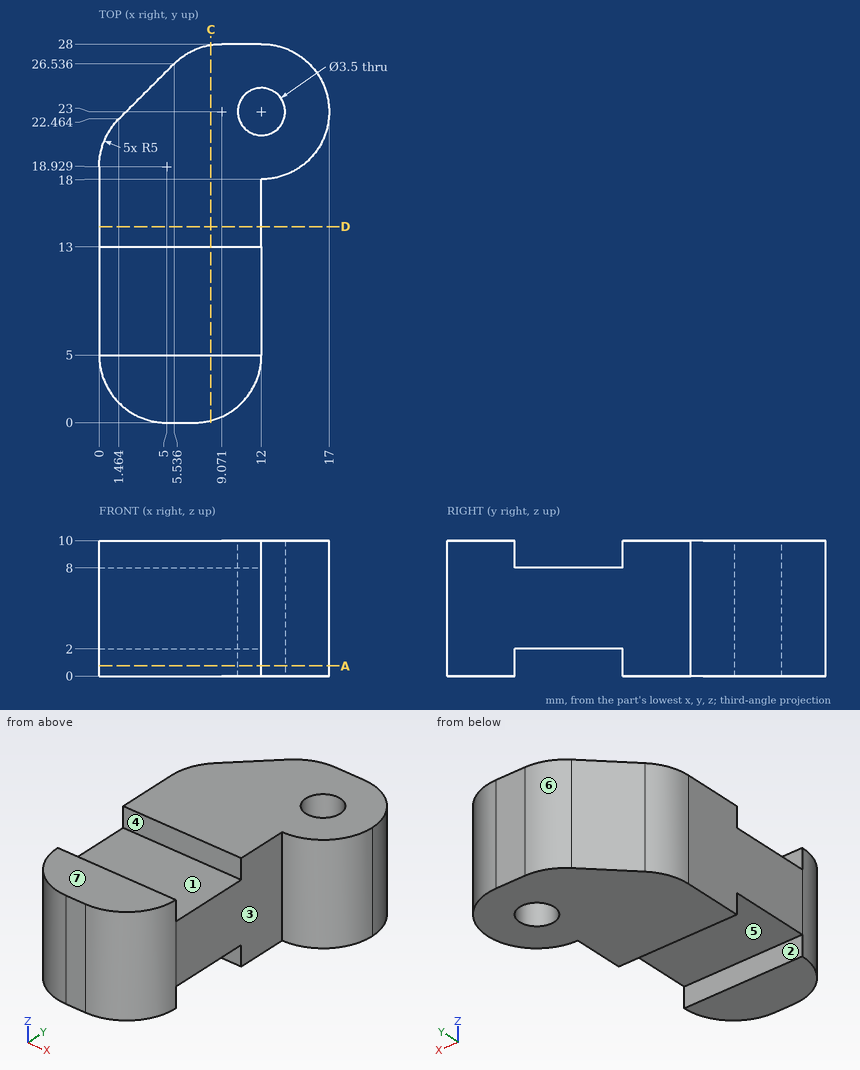
The figure shows three views and two pictorial views of one solid part (mm, origin at its lowest corner). Answer the questions. A direction names the side the tool comes from. Round coordinates to 2 decimals unless told otherwise and drop trailing zeros. Write each loop counter-clockwise with the first axis right and the second up, starting at its lowest first coordinate (ties: lowest second). Pieces come first, ordered by that corner, then holes. Notation, with made-up numbers: M 27.5,1.25 L 67.5,1.25 A35 ccw 67.5,39.25 Z; hole C -22,2.25 d4. An arc over 180 degrees is marked long. Use a Markdown table: item, result.
1) Consider line 1 (X direction, y = 10.25, z = 7.75); line 2 (Z direction, x = 6.25, y = 7.5); line 3 (X direction, y = 23.5, z = 7.25) (1 decimal). Determine where each line is inside the solid, lowest interval first. Write a range as [from, to].
Taken from the geometry:
| item | result |
|---|---|
| line 1 | x = [0, 12] |
| line 2 | z = [2, 8] |
| line 3 | x = [2.5, 10.3], [13.7, 17] |
2) The part is cut by section C-C on x = 8.25. Give the vertices of the cut face in (y, z).
Taken from the geometry:
| item | result |
|---|---|
| outline | M 0.16,0 L 5,0 L 5,2 L 13,2 L 13,0 L 27.93,0 L 27.93,10 L 13,10 L 13,8 L 5,8 L 5,10 L 0.16,10 Z |
3) Determine the mould class of the marked faces 4, 5, 6 and 7 for opening direction Y: pulls with the +Y half, pulls with the -Y half, needs draft (parallel to the pull), parting line crosses it, or undercut.
Taken from the geometry:
| item | result |
|---|---|
| face 4 | undercut |
| face 5 | undercut |
| face 6 | pulls with the +Y half |
| face 7 | needs draft |
4) The part is cut by section A-A on z = 0.75. State how many separate pieces and enclosed holes the cut face has, plus the area to 3 significant figures.
Taken from the geometry:
| item | result |
|---|---|
| separate pieces | 2 |
| enclosed holes | 1 |
| area | 233 mm2 |
5) The part is cut by section D-D on y = 14.5. Give the vertices of the cut face in (x, z), plus the area to 3 significant figures.
Taken from the geometry:
| item | result |
|---|---|
| outline | M 0,0 L 12,0 L 12,10 L 0,10 Z |
| area | 120 mm2 |
6) Which of the six approach directions +Z, -Z, +X, -X, +Y, -Y give full straight-line access (tool end or side, diameter ignored) to the marked faces 1, 2 and 3?
Taken from the geometry:
| item | result |
|---|---|
| face 1 | +Z, +X, -X |
| face 2 | -Z, +X, -X |
| face 3 | +Z, -Z, +X, -Y |
7) Flat-ended cylindrical pins translate along their axes: pin 1 (6 mm diameter, centred on y = 18.5, z = 6, fed in from +X); pin 2 (3 mm diameter, centred on y = 21, z = 4, fed in from +X) (1 decimal); pin 3 (2 mm diameter, centred on x = 5.5, z = 8.5, fed in from +Y). Find the tip coordinate at first contact, or state that the pin passes through.
Taken from the geometry:
| item | result |
|---|---|
| pin 1 | stops at x = 16.77 |
| pin 2 | stops at x = 17 |
| pin 3 | stops at y = 27.29 |
